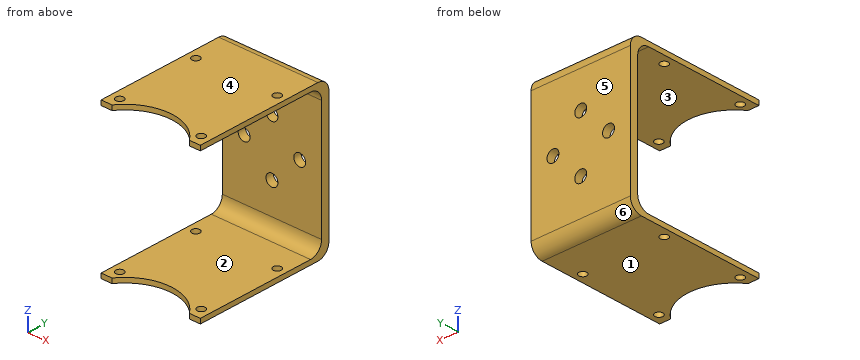
from build123d import *

# Parameters (mm, degrees)
EXTRUDE_1_DEPTH      = 2
SKETCH_4_W           = 25
SKETCH_4_H           = 1.2
EXTRUDE_3_DEPTH      = 40
FILLET_2_R           = 3
SKETCH_7_R           = 1
CUT_EXTRUDE_3_DEPTH  = 59.857879676
SKETCH_8_OUTSIDE_W   = 56.19
SKETCH_8_OUTSIDE_H   = 53.19
SKETCH_8_OUTSIDE_W_2 = 25
SKETCH_8_OUTSIDE_H_2 = 38
CUT_EXTRUDE_4_DEPTH  = 10
SKETCH_9_R           = 1.5
CUT_EXTRUDE_5_DEPTH  = 10


with BuildPart() as part:
    # 草图1 → 凸台-拉伸1 (new body)
    with BuildSketch(Plane(origin=(0, 0, 0), x_dir=(1, 0, 0), z_dir=(0, 1, 0))):
        Polygon((12.5, -10), (12.5, -19), (-12.5, -19), (-12.5, -10), (-20.5, -10), (-20.5, 10), (-12.5, 10), (-12.5, 19), (12.5, 19), (12.5, 10), (20.5, 10), (20.5, -10), align=None)
    extrude(amount=EXTRUDE_1_DEPTH)

    # 草图4 → 凸台-拉伸3 (add)
    with BuildSketch(Plane.XZ):
        with Locations((0, 18.4)):
            Rectangle(SKETCH_4_W, SKETCH_4_H)
        with Locations((0, -18.4)):
            Rectangle(SKETCH_4_W, SKETCH_4_H)
    extrude(amount=EXTRUDE_3_DEPTH)

    # 圆角2
    fillet_2_edges = [part.edges().sort_by_distance(p)[0] for p in [
        (0, 2, -19),
        (0, 2, 19),
        (0, 0, 17.8),
        (0, 0, -17.8),
    ]]
    fillet(fillet_2_edges, radius=FILLET_2_R)

    # 草图7 → 切除-拉伸3 (cut, through all)
    with BuildSketch(Plane.XY.offset(19)):
        with Locations((-10.25, -30.35)):
            Circle(SKETCH_7_R)
        with Locations((-10.25, -9.65)):
            Circle(SKETCH_7_R)
        with Locations((10.25, -9.65)):
            Circle(SKETCH_7_R)
        with Locations((10.25, -30.35)):
            Circle(SKETCH_7_R)
        with BuildLine():
            Line((-12.5, -33), (-9.746794345, -33))
            ThreePointArc((-9.746794345, -33), (0, -28), (9.746794345, -33))
            Line((9.746794345, -33), (12.5, -33))
            Line((12.5, -33), (12.5, -40))
            Line((12.5, -40), (-12.5, -40))
            Line((-12.5, -40), (-12.5, -33))
        make_face()
    extrude(amount=-CUT_EXTRUDE_3_DEPTH, mode=Mode.SUBTRACT)

    # 草图8 outside → 切除-拉伸4 (cut)
    with BuildSketch(Plane(origin=(0, 2, 0), x_dir=(1, 0, 0), z_dir=(0, 1, 0))):
        Rectangle(SKETCH_8_OUTSIDE_W, SKETCH_8_OUTSIDE_H)
        Rectangle(SKETCH_8_OUTSIDE_W_2, SKETCH_8_OUTSIDE_H_2, mode=Mode.SUBTRACT)
    extrude(amount=-CUT_EXTRUDE_4_DEPTH, mode=Mode.SUBTRACT)

    # 草图9 → 切除-拉伸5 (cut)
    with BuildSketch(Plane(origin=(0, 2, 0), x_dir=(1, 0, 0), z_dir=(0, 1, 0))):
        with Locations(Location((0, -7, 0), (0, 0, 270))):
            Circle(SKETCH_9_R)
        with Locations(Location((-7, 0, 0), (0, 0, 270))):
            Circle(SKETCH_9_R)
        with Locations(Location((0, 7, 0), (0, 0, 270))):
            Circle(SKETCH_9_R)
        with Locations(Location((7, 0, 0), (0, 0, 270))):
            Circle(SKETCH_9_R)
    extrude(amount=-CUT_EXTRUDE_5_DEPTH, mode=Mode.SUBTRACT)


solid = part.part
CAD build for the part. Positions are in the model's coordinates, mm. Face numbers are marked on the shaded views. A direction names the side the tool comes from. Round coordinates to 2 decimals unless told otherwise and drop trailing zeros. Loops run counter-clockwise (first coordinate to the right, second up) from the corner with the lowest first, then second, coordinate; pieces in that order, holes last.
(1) Cut at B-B (y = -24.5). Give the cut face in (x, z), plus the area to 3 significant figures.
(2) Cut at A-A (z = 7). Give the cut face in (x, y).
(3) Cut at C-C (x = 0). Give the cut face in (y, z).
(4) Wall check: line 1 along Z through (x, y) = (7.75, -18.5); line 2 along Y through (x, z) = (-10.25, 18.6); line 3 along X through (y, z) = (1.4, -7). Give the ranges that are in metal, low to high.
(5) Drop flat-ended pins along their axis: pin 1 (2.5 mm diameter, centred on x = 10.25, y = -30.35, fed in from +Z); pin 2 (2 mm diameter, centred on x = 7, z = -6.5, fed in from -Y). Give the stop position or say it passes through.
(6) Two-plate mould, pull along Z, no slides. Class the marked faces 3, 4, 5 and 6: +Z half, -Z half, draft (parallel to the pull), parting line (faces both ways), or undercut.
(7) Which spindle directions (+Z, -Z, +X, -X, +Y, -Y) get a long thin tool onto all of the face, cutting with end or side? Do the marked faces 1 and 2. Say none if no direction does.
(8) Cut at D-D (z = 0). Give the cut face in (x, y), plus the area to 3 significant figures.
Findings below:
1. outline: (-12.5, -19) - (12.5, -19) - (12.5, -17.8) - (-12.5, -17.8) - close; (-12.5, 17.8) - (12.5, 17.8) - (12.5, 19) - (-12.5, 19) - close
1. area: 60.0 mm2
2. outline: (-12.5, 0) - (-1.5, 0) - (-1.5, 2) - (-12.5, 2) - close; (1.5, 0) - (12.5, 0) - (12.5, 2) - (1.5, 2) - close
3. outline: (-28, -19) - (-1, -19) arc R3 ccw to (2, -16) - (2, -8.5) - (0, -8.5) - (0, -14.8) arc R3 cw to (-3, -17.8) - (-28, -17.8) - close; (-28, 17.8) - (-3, 17.8) arc R3 cw to (0, 14.8) - (0, 8.5) - (2, 8.5) - (2, 16) arc R3 ccw to (-1, 19) - (-28, 19) - close; (0, -5.5) - (2, -5.5) - (2, 5.5) - (0, 5.5) - close
4. line 1: z = -19 to -17.8, 17.8 to 19
4. line 2: y = -33 to -31.35, -29.35 to -10.65, -8.65 to 0.5
4. line 3: x = -12.5 to -1.5, 1.5 to 12.5
5. pin 1: stops at z = 19
5. pin 2: stops at y = 0
6. face 3: undercut
6. face 4: +Z half
6. face 5: draft
6. face 6: -Z half
7. face 1: -Z, +X, -X, +Y, -Y
7. face 2: +X, -X, -Y
8. outline: (-12.5, 0) - (-8.5, 0) - (-8.5, 2) - (-12.5, 2) - close; (-5.5, 0) - (5.5, 0) - (5.5, 2) - (-5.5, 2) - close; (8.5, 0) - (12.5, 0) - (12.5, 2) - (8.5, 2) - close
8. area: 38.0 mm2
